Here's the drawing with two shaded views (mm, measured from the low corner). I have some questions. Coordinates: 2 decimals unless noted, no trailing zeros. Order: outer loops, then holes, each group sorted by start corner. A loop starts at its lowest first (then second) coordinate and runs counter-clockwise, first axis right, second up. Notation, with made-up numbers: (-27, -35.5) - (12, -35.5) arc R22 cw to (12, -24.5) - close; hole circle Ø11 at (-9, -1.5). An arc over 180 degrees is marked (long way). Answer as CSV lines item,"result". Start each with the question number.
1. I want a section at C-C, the plane z = 6. List the corners of the cut face in (x, y) for me.
2. I need wall thicknesses on probe 1 along X at (y, z) = (2.5, 36); probe 2 along Z at (x, y) = (35.5, 0.4). Which ranges of each line are inside material? Lowest first, please.
3. I want a section at B-B, the plane y = 2.4. List the corners of the cut face in (x, z) for me, and give its area (3 significant figures).
4. I want a section at A-A, the plane x = 36. List the corners of the cut face in (y, z) for me.
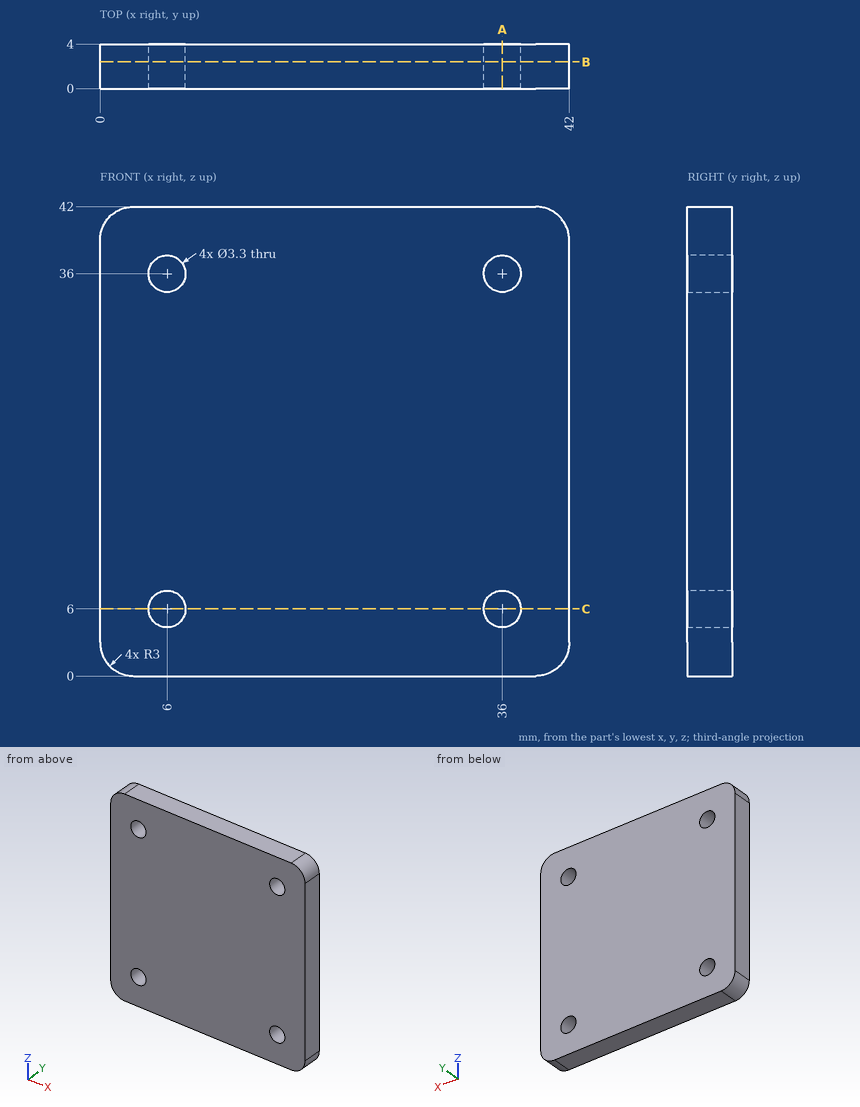
Solved:
1,outline,"(0, 0) - (4.35, 0) - (4.35, 4) - (0, 4) - close; (7.65, 0) - (34.35, 0) - (34.35, 4) - (7.65, 4) - close; (37.65, 0) - (42, 0) - (42, 4) - (37.65, 4) - close"
2,probe 1,"x = 0 to 4.35, 7.65 to 34.35, 37.65 to 42"
2,probe 2,"z = 0 to 4.43, 7.57 to 34.43, 37.57 to 42"
3,outline,"(0, 3) arc R3 ccw to (3, 0) - (39, 0) arc R3 ccw to (42, 3) - (42, 39) arc R3 ccw to (39, 42) - (3, 42) arc R3 ccw to (0, 39) - close; hole circle Ø3.3 at (6, 6); hole circle Ø3.3 at (6, 36); hole circle Ø3.3 at (36, 6); hole circle Ø3.3 at (36, 36)"
3,area,"1,720 mm2"
4,outline,"(0, 0) - (4, 0) - (4, 4.35) - (0, 4.35) - close; (0, 7.65) - (4, 7.65) - (4, 34.35) - (0, 34.35) - close; (0, 37.65) - (4, 37.65) - (4, 42) - (0, 42) - close"
